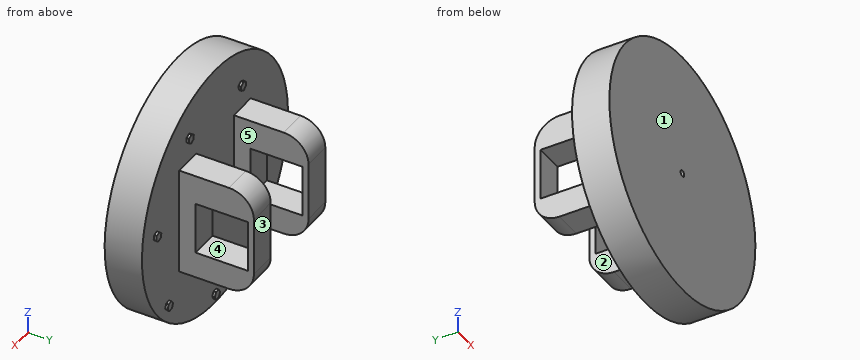
```python
from build123d import *

# Parameters (mm, degrees)
Y_KSEKLIK_EKSTR_ZYON1_DEPTH      = 10
Y_KSEKLIK_EKSTR_ZYON1_DEPTH_BACK = 20
IZIM1_R                          = 100
IZIM4_R                          = 2.55
KES_EKSTR_ZYON4_DEPTH            = 20.2
IZIM8_W                          = 23
IZIM8_H                          = 87
Y_KSEKLIK_EKSTR_ZYON5_DEPTH      = 70
KES_EKSTR_ZYON6_DEPTH            = 60
KES_EKSTR_ZYON6_DEPTH_BACK       = 60
IZIM9_W                          = 42
IZIM9_H                          = 42
Y_KSEKLIK_EKSTR_ZYON6_DEPTH      = 2
RADYUS1_R                        = 20


with BuildPart() as part:
    # Çizim1 → Yükseklik-Ekstrüzyon1 (new, two sides: drawn at the far end of the back side and taken through both)
    with BuildSketch(Plane(origin=(0, 0, 0), x_dir=(1, 0, 0), z_dir=(0, 1, 0)).offset(-Y_KSEKLIK_EKSTR_ZYON1_DEPTH_BACK)):
        with Locations(Location((0, 0, 0), (0, 0, 270))):
            Circle(IZIM1_R)
    extrude(amount=Y_KSEKLIK_EKSTR_ZYON1_DEPTH + Y_KSEKLIK_EKSTR_ZYON1_DEPTH_BACK)

    # Çizim4 → Kes-Ekstrüzyon4 (cut)
    with BuildSketch(Plane(origin=(0, 0, 0), x_dir=(1, 0, 0), z_dir=(0, 1, 0))):
        with Locations(Location((0, 0, 0), (0, 0, 270))):
            Circle(IZIM4_R)
    extrude(amount=-KES_EKSTR_ZYON4_DEPTH, mode=Mode.SUBTRACT)

    # Çizim8 → Yükseklik-Ekstrüzyon5 (add)
    with BuildSketch(Plane(origin=(0, 0, 0), x_dir=(1, 0, 0), z_dir=(0, 1, 0))):
        with Locations((-37.434640227, -1.29867582)):
            Rectangle(IZIM8_W, IZIM8_H)
        with Locations((37.434640227, -1.29867582)):
            Rectangle(IZIM8_W, IZIM8_H)
    extrude(amount=Y_KSEKLIK_EKSTR_ZYON5_DEPTH)

    # Çizim9 → Kes-Ekstrüzyon6 (cut, two sides: drawn at the far end of the back side and taken through both)
    with BuildSketch(Plane(origin=(0, 0, 0), x_dir=(0, 0, -1), z_dir=(1, 0, 0)).offset(-KES_EKSTR_ZYON6_DEPTH_BACK)):
        with Locations((0, 44.15078082)):
            Rectangle(IZIM9_W, IZIM9_H)
    extrude(amount=KES_EKSTR_ZYON6_DEPTH + KES_EKSTR_ZYON6_DEPTH_BACK, mode=Mode.SUBTRACT)

    # Çizim10 → Yükseklik-Ekstrüzyon6 (add)
    with BuildSketch(Plane(origin=(0, 10, 0), x_dir=(1, 0, 0), z_dir=(0, 1, 0))):
        Polygon((66.812616777, 58.515280774), (68.173954633, 61.983913061), (65.850699884, 64.897182371), (62.166107279, 64.341819393), (60.804769424, 60.873187106), (63.128024173, 57.959917797), align=None)
        Polygon((3.726211306, 92.48499002), (1.863105653, 95.711983671), (-1.863105653, 95.711983671), (-3.726211306, 92.48499002), (-1.863105653, 89.257996369), (1.863105653, 89.257996369), align=None)
        Polygon((79.587759086, -11.987424426), (83.148425279, -10.889104362), (83.977585299, -7.256316953), (81.246079126, -4.721849607), (77.685412933, -5.820169671), (76.856252913, -9.45295708), align=None)
        Polygon((32.431695509, -65.933150571), (35.510435771, -68.032200141), (38.867636153, -66.415457646), (39.146096273, -62.699665583), (36.06735601, -60.600616013), (32.710155628, -62.217358508), align=None)
        Polygon((-39.146096273, -62.699665583), (-38.867636153, -66.415457646), (-35.510435771, -68.032200141), (-32.431695509, -65.933150571), (-32.710155628, -62.217358508), (-36.06735601, -60.600616013), align=None)
        Polygon((-81.246079126, -4.721849607), (-83.977585299, -7.256316953), (-83.148425279, -10.889104362), (-79.587759086, -11.987424426), (-76.856252913, -9.45295708), (-77.685412933, -5.820169671), align=None)
        Polygon((-62.166107279, 64.341819393), (-65.850699884, 64.89718237), (-68.173954633, 61.983913061), (-66.812616777, 58.515280774), (-63.128024173, 57.959917797), (-60.804769424, 60.873187106), align=None)
    extrude(amount=Y_KSEKLIK_EKSTR_ZYON6_DEPTH)

    # Radyus1
    radyus1_edges = [part.edges().sort_by_distance(p)[0] for p in [
        (-37.434640227, 70, -42.20132418),
        (-37.434640227, 70, 44.79867582),
        (37.434640227, 70, -42.20132418),
        (37.434640227, 70, 44.79867582),
    ]]
    fillet(radyus1_edges, radius=RADYUS1_R)


solid = part.part
```
Verification items for the finished model (mm, model axes). Face numbers are marked on the shaded views. A direction names the side the tool comes from. Coordinates: 2 decimals unless noted, no trailing zeros. Write each loop counter-clockwise with the first axis right and the second up, starting at its lowest first coordinate (ties: lowest second). Pieces come first, ordered by that corner, then holes. Notation, with made-up numbers: M 38.25,-10 L 88.25,-10 A29 ccw 88.25,29 Z; hole C -39,44 d5. An arc over 180 degrees is marked long. One line per item, written item: value.
Item 1: Mould release check, pull along X, two halves, no side actions. Record for the marked faces 1 and 2: pulls with the +X half, pulls with the -X half, needs draft (parallel to the pull), parting line crosses it, or undercut.
Check sheet entries:
face 1: needs draft
face 2: undercut
Item 2: Section check C-C, the plane z = 0. Record the boundary of the cut face in (x, y), plus the area to 3 significant figures.
Check sheet entries:
outline: M -100,-20 L -2.55,-20 L -2.55,0 L 2.55,0 L 2.55,-20 L 100,-20 L 100,10 L 48.93,10 L 48.93,23.15 L 25.93,23.15 L 25.93,10 L -25.93,10 L -25.93,23.15 L -48.93,23.15 L -48.93,10 L -100,10 Z; M -48.93,65.15 L -25.93,65.15 L -25.93,70 L -48.93,70 Z; M 25.93,65.15 L 48.93,65.15 L 48.93,70 L 25.93,70 Z
area: 6,730 mm^2
Item 3: Section check A-A, the plane y = 38.5. Record the boundary of the cut face in (x, z), plus the area to 3 significant figures.
Check sheet entries:
outline: M -48.93,-42.2 L -25.93,-42.2 L -25.93,-21 L -48.93,-21 Z; M -48.93,21 L -25.93,21 L -25.93,44.8 L -48.93,44.8 Z; M 25.93,-42.2 L 48.93,-42.2 L 48.93,-21 L 25.93,-21 Z; M 25.93,21 L 48.93,21 L 48.93,44.8 L 25.93,44.8 Z
area: 2,070 mm^2
Item 4: Scan lines: line 1 along X through (y, z) = (16, 41.5); line 2 along X through (y, z) = (-8.75, 0); line 3 along Y through (x, z) = (37, -30.5). Record each from-to range of solid material in increasing order.
Check sheet entries:
line 1: x = -48.93 to -25.93, 25.93 to 48.93
line 2: x = -100 to -2.55, 2.55 to 100
line 3: y = -20 to 68.2
Item 5: Gauge pin test, flat ends, axial feed: pin 1 Ø8 at (y, z) = (-1.5, 70.5) entering from -X; pin 2 Ø1.5 at (y, z) = (42, -41.5) entering from -X; pin 3 Ø18.5 at (x, y) = (-35, 38) entering from -Z. Record the tip position at first contact, or that the pin passes through.
Check sheet entries:
pin 1: stops at x = -74.68
pin 2: stops at x = -48.93
pin 3: stops at z = -42.2
Item 6: Section check D-D, the plane x = 42. Record the boundary of the cut face in (y, z), plus the area to 3 significant figures.
Check sheet entries:
outline: M -20,-90.75 L 10,-90.75 L 10,-42.2 L 50,-42.2 A20 ccw 70,-22.2 L 70,24.8 A20 ccw 50,44.8 L 10,44.8 L 10,90.75 L -20,90.75 Z; hole M 23.15,-21 L 65.15,-21 L 65.15,21 L 23.15,21 Z
area: 8,730 mm^2
Item 7: Access from +Z, -Z, +X, -X, +Y, -Y to the whole of each face (thin tool, end or side, straight path). Record for the marked faces 3, 4 and 5.
Check sheet entries:
face 3: +Z, -Z, +X, -X, +Y
face 4: +X, -X
face 5: +Z, -Z, +Y
Item 8: Section check B-B, the plane y = 17. Record the boundary of the cut face in (x, z).
Check sheet entries:
outline: M -48.93,-42.2 L -25.93,-42.2 L -25.93,44.8 L -48.93,44.8 Z; M 25.93,-42.2 L 48.93,-42.2 L 48.93,44.8 L 25.93,44.8 Z
